Verification items for this drawing (mm, ordinates from the low corner). Round coordinates to 2 decimals unless told otherwise and drop trailing zeros. Order: outer loops, then holes, each group sorted by start corner. A loop starts at its lowest first (then second) coordinate and runs counter-clockwise, first axis right, second up. Notation, with made-up numbers: (83, -37.75) -> (111, -37.75) arc R21 ccw to (111, -16.75) -> close; hole circle Ø10 at (-23, 9). An arc over 180 degrees is marked (long way). Return JSON: item names as keys, results as strings. Group by question number.
Item 1: Sectioned sample at C-C on y = 20. Record the cut outline in (x, z) (1 decimal).
Item 2: Depth check by flat-ended pin: pin 1 Ø3.5 at (x, y) = (44, 35.31) entering from -Z. Enter the tip coordinate at first touch or a pass-through.
Item 3: Scan lines: probe 1 along Y at (x, z) = (44, 0.95); probe 2 along Y at (x, z) = (25.5, 1.15) (1 decimal); probe 3 along X at (y, z) = (24, 0.45) (1 decimal). Record each from-to range of solid material in increasing order. Write a range as from..to.
Item 4: Sectioned sample at B-B on x = 25.5. Record the cut outline in (y, z) (1 decimal).
Item 5: Sectioned sample at A-A on y = 35.31. Record the cut outline in (x, z).
Item 6: Sectioned sample at D-D on z = 1. Record the cut outline in (x, y) (1 decimal).
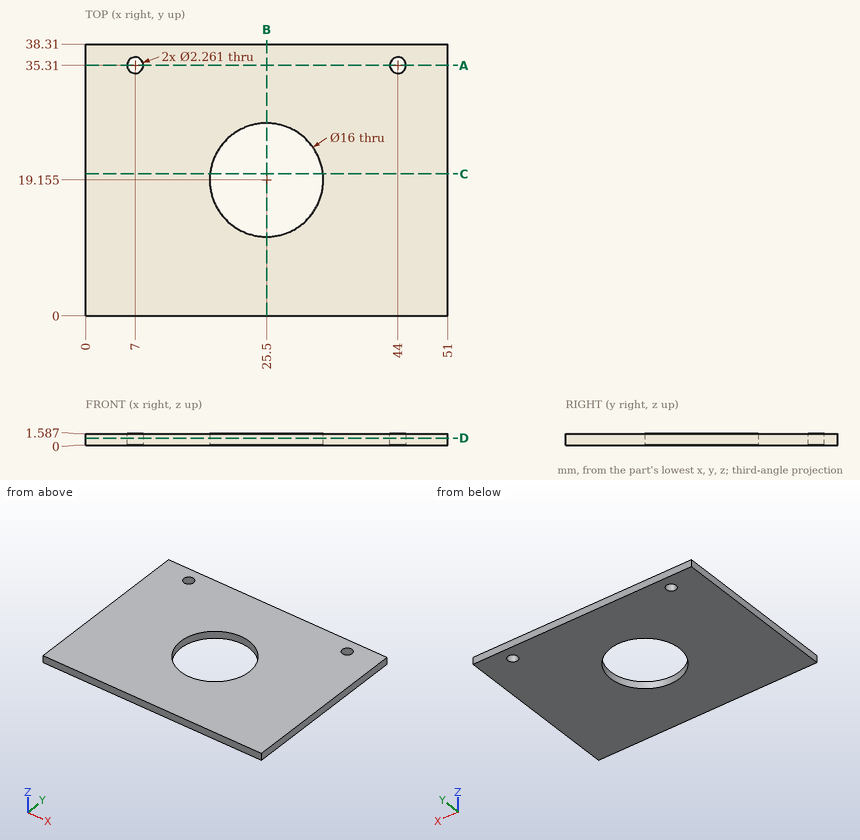
Recorded:
{
 "1": {"outline": "(0, 0) -> (17.5, 0) -> (17.5, 1.6) -> (0, 1.6) -> close; (33.5, 0) -> (51, 0) -> (51, 1.6) -> (33.5, 1.6) -> close"},
 "2": {"pin 1": "z = 0"},
 "3": {"probe 1": "0..34.18, 36.44..38.31", "probe 2": "0..11.2, 27.2..38.3", "probe 3": "0..19.1, 31.9..51"},
 "4": {"outline": "(0, 0) -> (11.2, 0) -> (11.2, 1.6) -> (0, 1.6) -> close; (27.2, 0) -> (38.3, 0) -> (38.3, 1.6) -> (27.2, 1.6) -> close"},
 "5": {"outline": "(0, 0) -> (5.87, 0) -> (5.87, 1.59) -> (0, 1.59) -> close; (8.13, 0) -> (42.87, 0) -> (42.87, 1.59) -> (8.13, 1.59) -> close; (45.13, 0) -> (51, 0) -> (51, 1.59) -> (45.13, 1.59) -> close"},
 "6": {"outline": "(0, 0) -> (51, 0) -> (51, 38.3) -> (0, 38.3) -> close; hole circle Ø2.3 at (7, 35.3); hole circle Ø16 at (25.5, 19.2); hole circle Ø2.3 at (44, 35.3)"}
}
